Model file for the job. Use its own axes, mm. Coordinates: 2 decimals unless noted, no trailing zeros. Write each loop counter-clockwise with the first axis right and the second up, starting at its lowest first coordinate (ties: lowest second). Pieces come first, ordered by that corner, then holes. Notation, with made-up numbers: M 4.25,-22.75 L 35.25,-22.75 A17 cw 35.25,10.25 Z; hole C 6,31 d11. An arc over 180 degrees is marked long. Put each result on its own line as item: value. Start each with the question number.
Q1. Cut at A-A (x = 0). Write the cut outline in (y, z).
Q2. Pull direction X, two halves, no side cores. Call faces 1 (the flat face through (0, -10, 0)), 2 (the cylindrical face through (13.281, -10.146, 0.986)), 3 (the cylindrical face through (22.4, -7.1, 1)), 4 (the cylindrical face through (-13.729, 6.728, 0.986)): pulls with the +X half, pulls with the -X half, needs draft (parallel to the pull), parting line crosses it, or undercut.
Q3. Drop a flat-ended pin along its axis: pin 1 (1 mm diameter, centred on y = -11.5, z = 0.5, fed in from -X). Give the stop position or say it passes through.
Q4. Cut at B-B (y = 0). Write the cut outline in (x, z).
Q5. Drill centre lines: line 1 along Y through (x, z) = (0, 1.15); line 2 along Y through (x, z) = (15.5, 1.95); line 3 along Y through (x, z) = (-16.5, 0.85). Where is each one in solid material? Low to high.
Q6. Cut at D-D (z = 1.4). Write the cut outline in (x, y) (3 decimals), then the cut area to 3 significant figures.
Q7. Cut at C-C (x = -5). Write the cut outline in (y, z) (3 decimals), then the cut area to 3 significant figures.
Autodesk Inventor part; units mm, degrees
ref_plane "YZ Plane" through (0, 0, 0) normal (1, 0, 0) x (0, 1, 0)
ref_plane "XZ Plane" through (0, 0, 0) normal (0, 1, 0) x (-1, 0, 0)
ref_plane "XY Plane" through (0, 0, 0) normal (0, 0, 1) x (1, 0, 0)
sketch "Sketch1" plane through (0, 0, 0) normal (0, 0, 1) x (1, 0, 0)
  circle A0 centre (0, 0) radius 23.5
  circle A1 centre (0, 0) radius 17.25
  circle A2 centre (0, 17.25) radius 2.25
  circle A3 centre (-14.9389, 8.625) radius 2.25
  circle A4 centre (-14.9389, -8.625) radius 2.25
  circle A5 centre (0, -17.25) radius 2.25
  circle A6 centre (14.9389, -8.625) radius 2.25
  circle A7 centre (14.9389, 8.625) radius 2.25
  circle A8 centre (0, 0) radius 8
  dimension "d1" = 34.5
  dimension "d0" = 47
  dimension "d2" = 4.5
  dimension "d5" = 360
  dimension "d7" = 16
extrude "Extrusion1" add sketch "Sketch1" along normal blind 2 contours A0 | A1 A6 A5 A4 A3 A2 A7
properties part number "rotor_hub_retainer"
Computed values:
1. outline: M -23.5,0 L -19.5,0 L -19.5,2 L -23.5,2 Z; M -15,0 L -8,0 L -8,2 L -15,2 Z; M 8,0 L 15,0 L 15,2 L 8,2 Z; M 19.5,0 L 23.5,0 L 23.5,2 L 19.5,2 Z
2. face 1: needs draft
2. face 2: undercut
2. face 3: parting line crosses it
2. face 4: undercut
3. pin 1: x = -20.77
4. outline: M -23.5,0 L -8,0 L -8,2 L -23.5,2 Z; M 8,0 L 23.5,0 L 23.5,2 L 8,2 Z
5. line 1: -23.5 to -19.5, -15 to -8, 8 to 15, 19.5 to 23.5
5. line 2: -17.66 to -10.8, -6.45 to 6.45, 10.8 to 17.66
5. line 3: -16.73 to -10.25, -7 to 7, 10.25 to 16.73
6. outline: C 0,0 d47; hole C -14.939,-8.625 d4.5; hole C -14.939,8.625 d4.5; hole C 0,0 d16; hole C 0,-17.25 d4.5; hole C 0,17.25 d4.5; hole C 14.939,-8.625 d4.5; hole C 14.939,8.625 d4.5
6. area: 1,440 mm2
7. outline: M -22.962,0 L -6.245,0 L -6.245,2 L -22.962,2 Z; M 6.245,0 L 22.962,0 L 22.962,2 L 6.245,2 Z
7. area: 66.9 mm2
